The model under review builds one solid part; all positions refer to its coordinate system, in mm. Face numbers are marked on the shaded views. A direction names the side the tool comes from. Give positions to 0.01 mm unless a question says otherwise; leave off trailing zeros. Order: outer loops, then holes, each group sorted by start corner. A loop starts at its lowest first (then second) coordinate and runs counter-clockwise, first axis right, second up. Notation, with made-up numbers: (2.25, 61.5) - (53.25, 61.5) arc R29 cw to (53.25, 85.5) - close; hole circle Ø4 at (-13.75, 22). An arc over 180 degrees is marked (long way). Use a Markdown table: item, result. Add a question column.
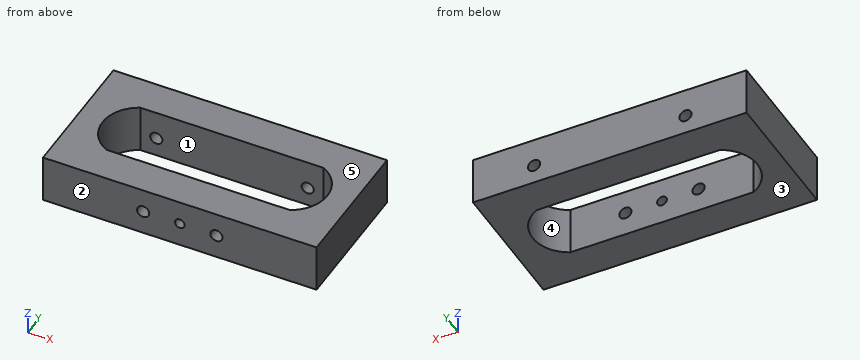
```python
from build123d import *

# Parameters (mm, degrees)
SKIZZE1_W                       = 56
SKIZZE1_H                       = 28
AUFSATZ_LINEAR_AUSTRAGEN1_DEPTH = 10
SCHNITT_LINEAR_AUSTRAGEN1_DEPTH = 33.86335345
KERNLOCH_F_R_M3_GEWINDE1_D      = 2.5
KERNLOCH_F_R_M3_GEWINDE1_DEPTH  = 8.5
KERNLOCH_F_R_M3_GEWINDE1_TIP    = 0.751075774
KERNLOCH_F_R_M3_GEWINDE2_D      = 2.5
KERNLOCH_F_R_M3_GEWINDE2_DEPTH  = 7.25
F_2_0MM_STIFTLOCH1_D            = 2
F_2_0MM_STIFTLOCH1_DEPTH        = 8.5
F_2_0MM_STIFTLOCH1_TIP          = 0.600860619


with BuildPart() as part:
    # Skizze1 → Aufsatz-Linear austragen1 (new body)
    with BuildSketch(Plane.XY):
        Rectangle(SKIZZE1_W, SKIZZE1_H)
    extrude(amount=AUFSATZ_LINEAR_AUSTRAGEN1_DEPTH)

    # Skizze2 → Schnitt-Linear austragen1 (cut, through all)
    with BuildSketch(Plane(origin=(0, 0, 0), x_dir=(-1, 0, 0), z_dir=(0, 0, -1))):
        with BuildLine():
            Line((-18.769174208, 6.75), (18.769174208, 6.75))
            ThreePointArc((18.769174208, 6.75), (23, 0), (18.769174208, -6.75))
            Line((18.769174208, -6.75), (-18.769174208, -6.75))
            ThreePointArc((-18.769174208, -6.75), (-23, 0), (-18.769174208, 6.75))
        make_face()
    extrude(amount=-SCHNITT_LINEAR_AUSTRAGEN1_DEPTH, mode=Mode.SUBTRACT)

    # Kernloch für M3 Gewinde1
    with Locations(Plane(origin=(0, -14, 0), x_dir=(-1, 0, 0), z_dir=(0, -1, 0))):
        with Locations((-7.5, -5), (7.5, -5)):
            Hole(KERNLOCH_F_R_M3_GEWINDE1_D / 2, depth=KERNLOCH_F_R_M3_GEWINDE1_DEPTH)
            with Locations((0, 0, -(KERNLOCH_F_R_M3_GEWINDE1_DEPTH + KERNLOCH_F_R_M3_GEWINDE1_TIP / 2))):  # 118° drill point
                Cone(0, KERNLOCH_F_R_M3_GEWINDE1_D / 2, KERNLOCH_F_R_M3_GEWINDE1_TIP, mode=Mode.SUBTRACT)

    # Kernloch für M3 Gewinde2
    with Locations(Plane(origin=(0, 14, 0), x_dir=(1, 0, 0), z_dir=(0, 1, 0))):
        with Locations((15.5, -4), (-15.5, -4)):
            Hole(KERNLOCH_F_R_M3_GEWINDE2_D / 2, depth=KERNLOCH_F_R_M3_GEWINDE2_DEPTH)

    # Ø2.0mm Stiftloch1
    with Locations(Plane(origin=(0, -14, 0), x_dir=(-1, 0, 0), z_dir=(0, -1, 0))):
        with Locations((0, -5)):
            Hole(F_2_0MM_STIFTLOCH1_D / 2, depth=F_2_0MM_STIFTLOCH1_DEPTH)
            with Locations((0, 0, -(F_2_0MM_STIFTLOCH1_DEPTH + F_2_0MM_STIFTLOCH1_TIP / 2))):  # 118° drill point
                Cone(0, F_2_0MM_STIFTLOCH1_D / 2, F_2_0MM_STIFTLOCH1_TIP, mode=Mode.SUBTRACT)


solid = part.part
```
Q1. We need section D-D (x = 19.5). Write out the cut boundary in (y, z).
Q2. Wall thickness on probe 1 along X at (y, z) = (-12, 5); probe 2 along X at (y, z) = (11.25, 4); probe 3 along Y at (x, z) = (11, 1.5): over which ranges is each line inside the solid? List them lowest first.
Q3. Machinability: for the marked faces 4 and 5, which of the approach directions +Z, -Z, +X, -X, +Y, -Y give a long, thin tool a straight path to every point of the face, cutting with its end or side? Answer none if there is none.
Q4. We need section A-A (y = -6). Write out the cut boundary in (x, z).
Q5. We need section C-C (x = 7.5). Write out the cut boundary in (y, z).
Q6. We need section B-B (z = 7). Write out the cut boundary in (x, y).
Q7. Draft analysis for pull direction Y (two halves, no side actions). For the marked faces 1, 2 and 3, state which applies: pulls with the +Y half, pulls with the -Y half, needs draft (parallel to the pull), parting line crosses it, or undercut.
Here are the results:
| question | item | result |
|---|---|---|
| 1 | outline | (-14, 0) - (-6.34, 0) - (-6.34, 10) - (-14, 10) - close; (6.34, 0) - (14, 0) - (14, 10) - (6.34, 10) - close |
| 2 | probe 1 | -28 to -8.75, -6.25 to -1, 1 to 6.25, 8.75 to 28 |
| 2 | probe 2 | -28 to -16.75, -14.25 to 14.25, 16.75 to 28 |
| 2 | probe 3 | -14 to -6.75, 6.75 to 14 |
| 3 | face 4 | +Z, -Z |
| 3 | face 5 | +Z, +X, -X, +Y, -Y |
| 4 | outline | (-28, 0) - (-20, 0) - (-20, 10) - (-28, 10) - close; (20, 0) - (28, 0) - (28, 10) - (20, 10) - close |
| 5 | outline | (-14, 0) - (-6.75, 0) - (-6.75, 3.75) - (-14, 3.75) - close; (-14, 6.25) - (-6.75, 6.25) - (-6.75, 10) - (-14, 10) - close; (6.75, 0) - (14, 0) - (14, 10) - (6.75, 10) - close |
| 6 | outline | (-28, -14) - (28, -14) - (28, 14) - (-28, 14) - close; hole (-18.77, -6.75) - (18.77, -6.75) arc R7.5 ccw to (18.77, 6.75) - (-18.77, 6.75) arc R7.5 ccw to start |
| 7 | face 1 | undercut |
| 7 | face 2 | pulls with the -Y half |
| 7 | face 3 | needs draft |
